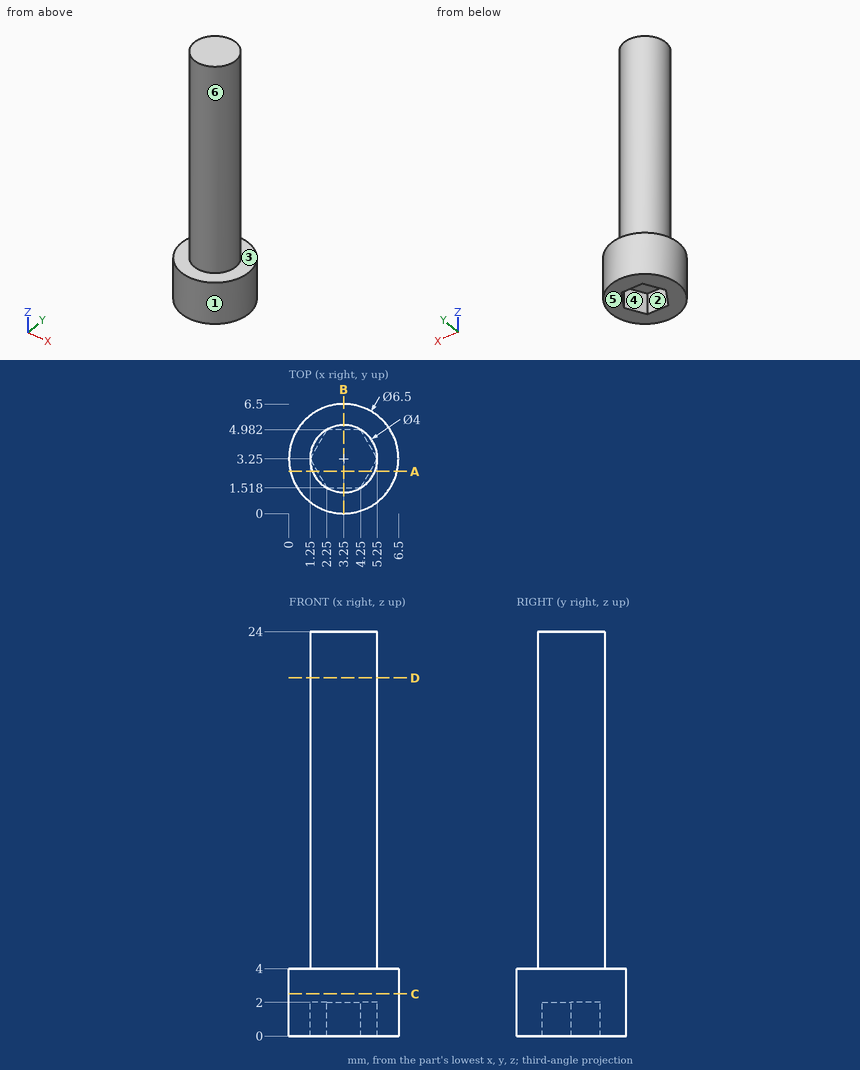
Source: three-view drawing plus pictorial views. Frame: mm from the lowest corner of the part. A direction names the side the tool comes from. Round coordinates to 2 decimals unless told otherwise and drop trailing zeros. Loops run counter-clockwise (first coordinate to the right, second up) from the corner with the lowest first, then second, coordinate; pieces in that order, holes last. Notation, with made-up numbers: (15.25, 34) - (51.25, 34) arc R27 cw to (51.25, 72) - close; hole circle Ø4 at (10, 18.5). An arc over 180 degrees is marked (long way). Write each question's results on one line, items separated by ' | '. Start each with the question number.
1) Cut plane A-A on y = 2.5. Return loops of the section in (x, z), then the cut area to 3 significant figures.
2) Cut plane D-D on z = 21.25. Return loops of the section in (x, y), then the cut area to 3 significant figures.
3) Cut plane C-C on z = 2.5. Return loops of the section in (x, y), then the cut area to 3 significant figures.
4) First-contact query: P1, Ø1, axis at x = 1.5, z = 11, coming from the +Y side; P2, Ø1.5, axis at y = 1.5, z = 4.5, coming from the +X side; P3, Ø3, axis at x = 3, z = 11, coming from the -Y side. Flat tips, straight axial feed; report the tip coordinate or a pass-through.
5) Cut plane B-B on x = 3.25. Return loops of the section in (y, z), then the cut area to 3 significant figures.
6) Access query for the marked faces 4, 5 and 6. Directions: +Z, -Z, +X, -X, +Y, -Y. A direction counts if a zero-diameter tool reaches every point of the face in a straight line with its end or side. Return the directions, or none.
7) Mould query, pull axis X, two halves, no side actions, for the marked faces 1, 2 and 3. Classes: released by +X, released by -X, zero draft, split by the parting line, or undercut.
8) Line query: probe 1 along Z at (x, y) = (3.5, 3.25); probe 2 along Z at (x, y) = (3, 0.5); probe 3 along X at (y, z) = (2.5, 1). Output: solid intervals per line, ascending. Write a range as [from, to].
Verdict:
1) outline: (0.09, 0) - (1.68, 0) - (1.68, 2) - (4.82, 2) - (4.82, 0) - (6.41, 0) - (6.41, 4) - (5.1, 4) - (5.1, 24) - (1.4, 24) - (1.4, 4) - (0.09, 4) - close | area: 93.2 mm2
2) outline: circle Ø4 at (3.25, 3.25) | area: 12.6 mm2
3) outline: circle Ø6.5 at (3.25, 3.25) | area: 33.2 mm2
4) P1: stops at y = 4.81 | P2: stops at x = 6.27 | P3: stops at y = 1.25
5) outline: (0, 0) - (1.52, 0) - (1.52, 2) - (4.98, 2) - (4.98, 0) - (6.5, 0) - (6.5, 4) - (5.25, 4) - (5.25, 24) - (1.25, 24) - (1.25, 4) - (0, 4) - close | area: 99.1 mm2
6) face 4: -Z | face 5: -Z, +X, -X, +Y, -Y | face 6: +Z
7) face 1: split by the parting line | face 2: undercut | face 3: zero draft
8) probe 1: z = [2, 24] | probe 2: z = [0, 4] | probe 3: x = [0.09, 1.68], [4.82, 6.41]
